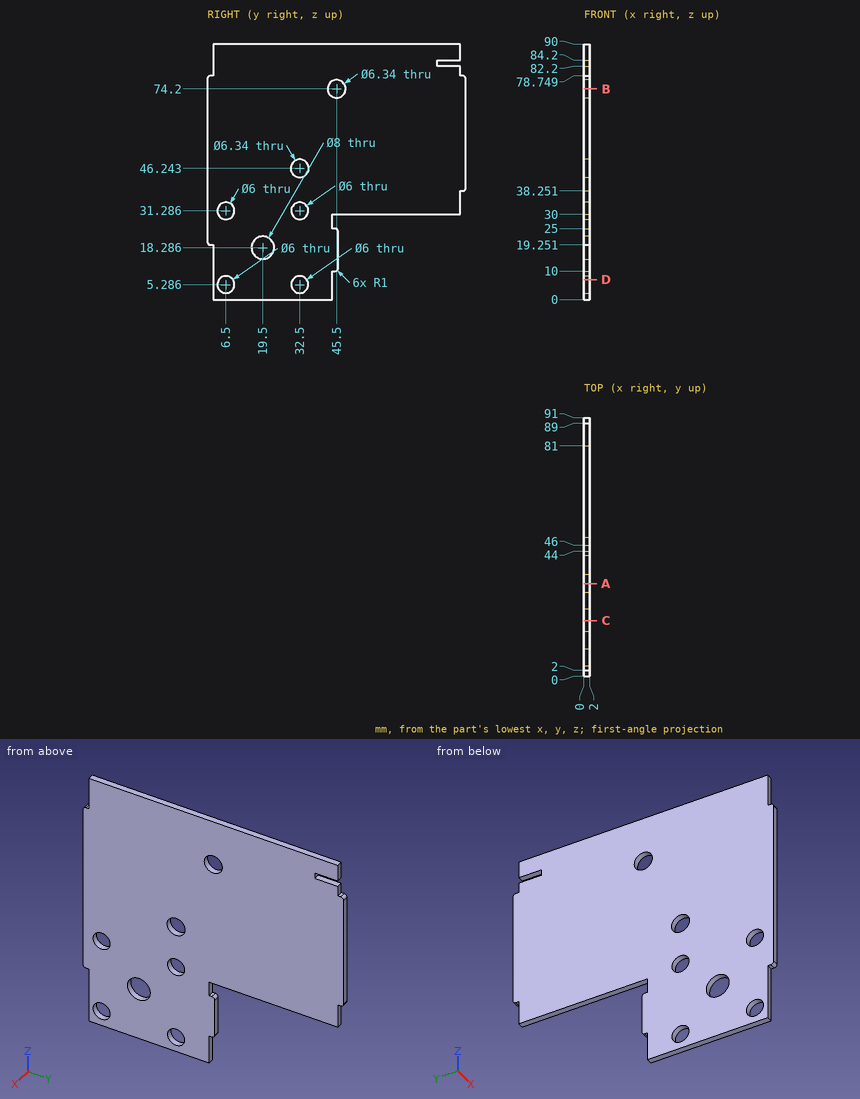
Geometry check sheet. Reference: drawing and pictorial views, mm from the part's lowest x, y, z. Coordinates: 2 decimals unless noted, no trailing zeros. Order: outer loops, then holes, each group sorted by start corner. A loop starts at its lowest first (then second) coordinate and runs counter-clockwise, first axis right, second up.
1. Sectioned sample at C-C, the plane y = 19.5. Record the cut outline in (x, z) (1 decimal).
Results found:
outline: (0, 0) - (2, 0) - (2, 14.3) - (0, 14.3) - close; (0, 22.3) - (2, 22.3) - (2, 90) - (0, 90) - close
2. Sectioned sample at B-B, the plane z = 74.2. Record the cut outline in (x, y).
Results found:
outline: (0, 0) - (2, 0) - (2, 42.33) - (0, 42.33) - close; (0, 48.67) - (2, 48.67) - (2, 91) - (0, 91) - close
3. Go/stop test with flat-tipped pins: pin 1 Ø1 at (x, z) = (1, 26.5) entering from +Y; pin 2 Ø0.8 at (x, y) = (1, 89.5) entering from -Z; pin 3 Ø0.6 at (x, z) = (0.5, 88) entering from +Y. Record where each tip stops, or that it passes through.
Results found:
pin 1: stops at y = 44
pin 2: stops at z = 38.25
pin 3: stops at y = 89
4. Scan lines: line 1 (Z direction, x = 1.5, y = 35) (1 decimal); line 2 (Z direction, x = 1.45, y = 83); line 3 (Y direction, x = 0.55, z = 18.5) (1 decimal). Record each from-to range of solid material in increasing order.
Results found:
line 1: z = 0 to 3.6, 6.9 to 29.6, 32.9 to 44.3, 48.2 to 90
line 2: z = 30 to 82.2, 84.2 to 90
line 3: y = 2 to 15.5, 23.5 to 46
5. Sectioned sample at D-D, the plane z = 7. Record the cut outline in (x, y).
Results found:
outline: (0, 2) - (2, 2) - (2, 4.04) - (0, 4.04) - close; (0, 8.96) - (2, 8.96) - (2, 30.04) - (0, 30.04) - close; (0, 34.96) - (2, 34.96) - (2, 44) - (0, 44) - close
6. Sectioned sample at A-A, the plane y = 32.5. Record the cut outline in (x, z) (1 decimal).
Results found:
outline: (0, 0) - (2, 0) - (2, 2.3) - (0, 2.3) - close; (0, 8.3) - (2, 8.3) - (2, 28.3) - (0, 28.3) - close; (0, 34.3) - (2, 34.3) - (2, 43.1) - (0, 43.1) - close; (0, 49.4) - (2, 49.4) - (2, 90) - (0, 90) - close
